Verification items for this drawing (mm, ordinates from the low corner). Round coordinates to 2 decimals unless told otherwise and drop trailing zeros. Order: outer loops, then holes, each group sorted by start corner. A loop starts at its lowest first (then second) coordinate and runs counter-clockwise, first axis right, second up. Notation, with made-up numbers: M -22,83.25 L 31,83.25 A29 cw 31,119.25 Z; hole C 20.5,63.25 d7. An arc over 180 degrees is marked long. Return JSON: item names as keys, results as strings. Group by question number.
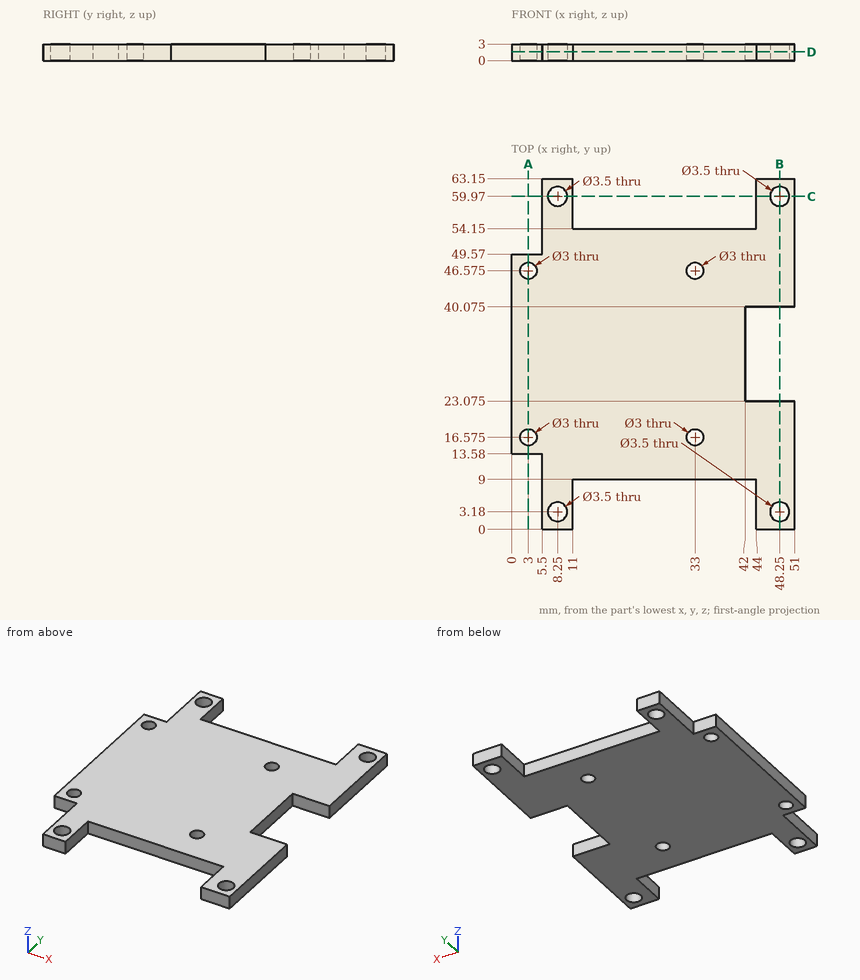
1. Cross-section at C-C (y = 59.97). Enter the section's corners in (x, z), plus the area to 3 significant figures.
2. Go/stop test with flat-tipped pins: pin 1 (3 mm diameter, centred on x = 48.25, y = 59.97, fed in from -Z); pin 2 (1.5 mm diameter, centred on x = 4, z = 2, fed in from -Y); pin 3 (1 mm diameter, centred on x = 36, z = 1, fed in from -Y); pin 4 (1.5 mm diameter, centred on y = 27.5, z = 1, fed in from +X). Record where each tip stops, or that it passes through.
3. Cross-section at B-B (x = 48.25). Enter the section's corners in (y, z) (3 decimals).
4. Thickness scan on line 1 along Y through (x, z) = (8.25, 1.15); line 2 along Y through (x, z) = (3, 0.95) (3 decimals); line 3 along Y through (x, z) = (48.25, 1.7) (3 decimals). Record the ranges inside material, lowest first. Write a range as from..to.
5. Cross-section at A-A (x = 3). Enter the section's corners in (y, z) (3 decimals).
6. Cross-section at D-D (z = 1.6). Give the number of separate pieces and of enclosed holes in the cut face, plus the area to 3 significant figures.
Computed:
{
 "1": {"outline": "M 5.5,0 L 6.5,0 L 6.5,3 L 5.5,3 Z; M 10,0 L 11,0 L 11,3 L 10,3 Z; M 44,0 L 46.5,0 L 46.5,3 L 44,3 Z; M 50,0 L 51,0 L 51,3 L 50,3 Z", "area": "16.5 mm²"},
 "2": {"pin 1": "passes through", "pin 2": "stops at y = 13.58", "pin 3": "stops at y = 9", "pin 4": "stops at x = 42"},
 "3": {"outline": "M 0,0 L 1.43,0 L 1.43,3 L 0,3 Z; M 4.93,0 L 23.075,0 L 23.075,3 L 4.93,3 Z; M 40.075,0 L 58.22,0 L 58.22,3 L 40.075,3 Z; M 61.72,0 L 63.15,0 L 63.15,3 L 61.72,3 Z"},
 "4": {"line 1": "y = 0..1.43, 4.93..58.22, 61.72..63.15", "line 2": "y = 13.58..15.075, 18.075..45.075, 48.075..49.57", "line 3": "y = 0..1.43, 4.93..23.075, 40.075..58.22, 61.72..63.15"},
 "5": {"outline": "M 13.58,0 L 15.075,0 L 15.075,3 L 13.58,3 Z; M 18.075,0 L 45.075,0 L 45.075,3 L 18.075,3 Z; M 48.075,0 L 49.57,0 L 49.57,3 L 48.075,3 Z"},
 "6": {"separate pieces": "1", "enclosed holes": "8", "area": "2,260 mm²"}
}
